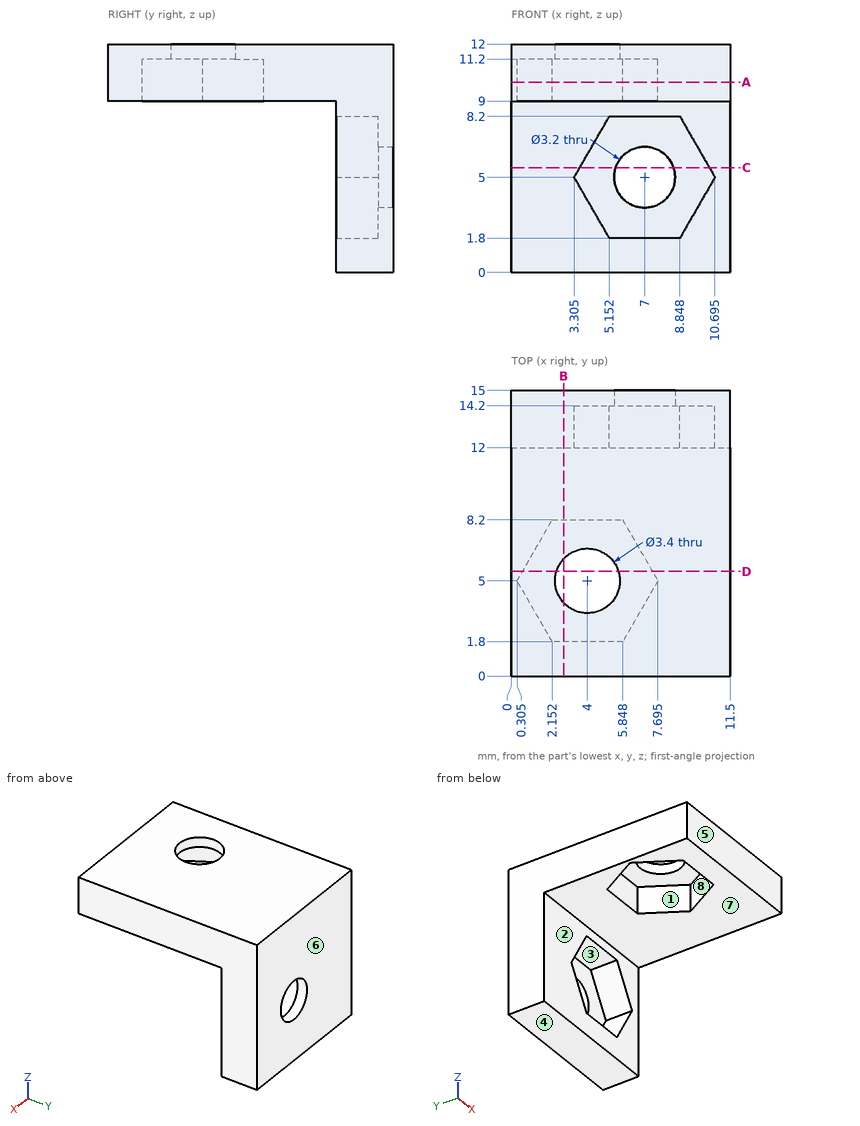
The figure shows three views and two pictorial views of one solid part (mm, origin at its lowest corner). Answer the questions. A direction names the side the tool comes from. Give positions to 0.01 mm unless a question says otherwise; leave off trailing zeros. Order: outer loops, then holes, each group sorted by start corner. A loop starts at its lowest first (then second) coordinate and runs counter-clockwise, first axis right, second up. Notation, with made-up numbers: M -18.5,55 L 4.5,55 A13 ccw 4.5,62 Z; hole C 45,58 d9. An arc over 180 degrees is marked long. Return JSON: item names as keys, results as strings.
Q1. Find section D-D, the plane y = 5.5. Write down the section's boundary in (x, z) (1 decimal), and give its area (3 significant figures).
Answer below:
{"outline": "M 0,9 L 0.6,9 L 0.6,11.2 L 2.4,11.2 L 2.4,12 L 0,12 Z; M 5.6,11.2 L 7.4,11.2 L 7.4,9 L 11.5,9 L 11.5,12 L 5.6,12 Z", "area": "16.9 mm^2"}
Q2. Find section B-B, the plane x = 2.75. Write down the section's boundary in (y, z).
Answer below:
{"outline": "M 0,9 L 1.8,9 L 1.8,11.2 L 3.85,11.2 L 3.85,12 L 0,12 Z; M 6.15,11.2 L 8.2,11.2 L 8.2,9 L 12,9 L 12,0 L 15,0 L 15,12 L 6.15,12 Z"}
Q3. Find section C-C, the plane z = 5.5. Write down the section's boundary in (x, y).
Answer below:
{"outline": "M 0,12 L 3.59,12 L 3.59,14.2 L 5.48,14.2 L 5.48,15 L 0,15 Z; M 8.52,14.2 L 10.41,14.2 L 10.41,12 L 11.5,12 L 11.5,15 L 8.52,15 Z"}
Q4. Each of these flat-tipped pins is pushed along its axis until it touches: pin 1 (3 mm diameter, centred on x = 7, z = 5, fed in from +Y); pin 2 (1.9 mm diameter, centred on x = 3, y = 5.5, fed in from -Z); pin 3 (2.5 mm diameter, centred on x = 4.5, z = 3.5, fed in from -Y); pin 4 (1.9 mm diameter, centred on x = 6.5, z = 3.5, fed in from -Y). Where does it stop, or does it pass through?
Answer below:
{"pin 1": "passes through", "pin 2": "stops at z = 11.2", "pin 3": "stops at y = 12", "pin 4": "stops at y = 14.2"}
Q5. Which of the six approach directions +Z, -Z, +X, -X, +Y, -Y give full straight-line access (tool end or side, diameter ignored) to the marked faces 1, 2, 3 and 4?
Answer below:
{"face 1": "-Z", "face 2": "-Z, +X, -X, -Y", "face 3": "-Y", "face 4": "-Z, +X, -X, +Y, -Y"}
Q6. The mould has two halves that part along Y. Classify the marked faces 5, 6, 7 and 8: pulls with the +Y half, pulls with the -Y half, needs draft (parallel to the pull), parting line crosses it, or undercut.
Answer below:
{"face 5": "pulls with the -Y half", "face 6": "pulls with the +Y half", "face 7": "needs draft", "face 8": "undercut"}
Q7. Find section A-A, the plane z = 10. Write down the section's boundary in (x, y) (1 decimal), and give its area (3 significant figures).
Answer below:
{"outline": "M 0,0 L 11.5,0 L 11.5,15 L 0,15 Z; hole M 0.3,5 L 2.2,1.8 L 5.8,1.8 L 7.7,5 L 5.8,8.2 L 2.2,8.2 Z", "area": "137 mm^2"}
Q8. Find the intervals of material crossed by line 1 along Y through (x, z) = (4, 11.6); line 2 along X through (y, z) = (14.6, 5); line 3 along Z through (x, y) = (7, 14.4), in increasing order. Write a range as [from, to].
Answer below:
{"line 1": "y = [0, 3.3], [6.7, 15]", "line 2": "x = [0, 5.4], [8.6, 11.5]", "line 3": "z = [0, 3.4], [6.6, 12]"}
